Verification items for this drawing (mm, ordinates from the low corner). A direction names the side the tool comes from. Coordinates: 2 decimals unless noted, no trailing zeros. Write each loop counter-clockwise with the first axis right and the second up, starting at its lowest first coordinate (ties: lowest second). Pieces come first, ordered by that corner, then holes. Notation, with made-up numbers: (16.5, 65.5) -> (71.5, 65.5) arc R21 ccw to (71.5, 97.5) -> close; hole circle Ø2 at (30.25, 28). An arc over 180 degrees is marked (long way). Put each result on its own line as item: value. Start each with the question number.
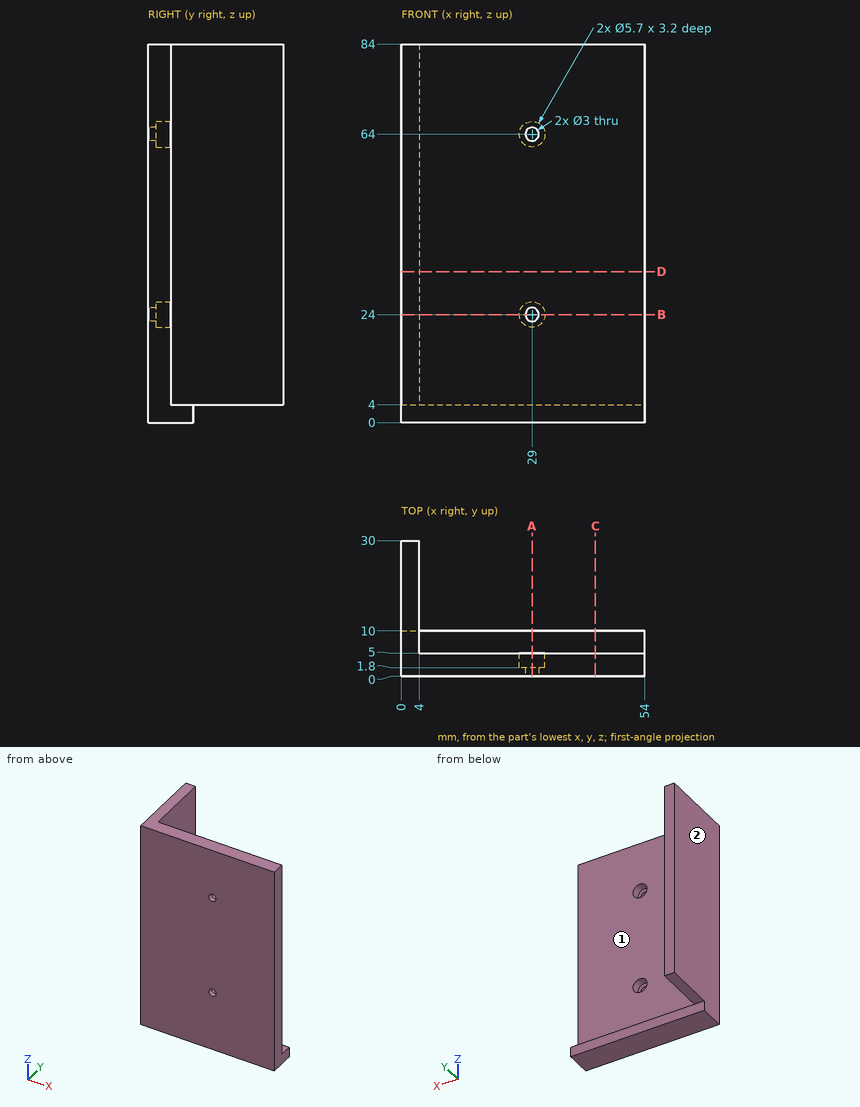
Item 1: Section check B-B, the plane z = 24. Enter the section's corners in (x, y), and give its area (3 significant figures).
Item 2: Section check A-A, the plane x = 29. Enter the section's corners in (y, z).
Item 3: Scan lines: line 1 along Z through (x, y) = (29, 3.7); line 2 along Z through (x, y) = (29, 0.75); line 3 along X through (y, z) = (0.4, 64). Record each from-to range of solid material in increasing order. Write a range as [from, to].
Item 4: Go/stop test with flat-tipped pins: P1, Ø10, axis at x = 10, z = 66.5, coming from the +Y side; P2, Ø3, axis at x = 21, z = 2, coming from the +Y side; P3, Ø3, axis at x = 2.5, y = 18.5, coming from the -Z side. Record where each tip stops, or that it passes through.
Item 5: Section check D-D, the plane z = 33.5. Enter the section's corners in (x, y), and give its area (3 significant figures).
Item 6: Section check C-C, the plane x = 43. Enter the section's corners in (y, z).
Item 7: Access from +Z, -Z, +X, -X, +Y, -Y to the whole of each face (thin tool, end or side, straight path). Record for the marked faces 1 and 2.
From the geometry:
1. outline: (0, 0) -> (27.5, 0) -> (27.5, 1.8) -> (26.15, 1.8) -> (26.15, 5) -> (4, 5) -> (4, 30) -> (0, 30) -> close; (30.5, 0) -> (54, 0) -> (54, 5) -> (31.85, 5) -> (31.85, 1.8) -> (30.5, 1.8) -> close
1. area: 346 mm²
2. outline: (0, 0) -> (10, 0) -> (10, 4) -> (5, 4) -> (5, 21.15) -> (1.8, 21.15) -> (1.8, 22.5) -> (0, 22.5) -> close; (0, 25.5) -> (1.8, 25.5) -> (1.8, 26.85) -> (5, 26.85) -> (5, 61.15) -> (1.8, 61.15) -> (1.8, 62.5) -> (0, 62.5) -> close; (0, 65.5) -> (1.8, 65.5) -> (1.8, 66.85) -> (5, 66.85) -> (5, 84) -> (0, 84) -> close
3. line 1: [0, 21.15], [26.85, 61.15], [66.85, 84]
3. line 2: [0, 22.5], [25.5, 62.5], [65.5, 84]
3. line 3: [0, 27.5], [30.5, 54]
4. P1: y = 5
4. P2: y = 10
4. P3: z = 4
5. outline: (0, 0) -> (54, 0) -> (54, 5) -> (4, 5) -> (4, 30) -> (0, 30) -> close
5. area: 370 mm²
6. outline: (0, 0) -> (10, 0) -> (10, 4) -> (5, 4) -> (5, 84) -> (0, 84) -> close
7. face 1: +Z, +X, +Y
7. face 2: +Z, -Z, -X, +Y, -Y
